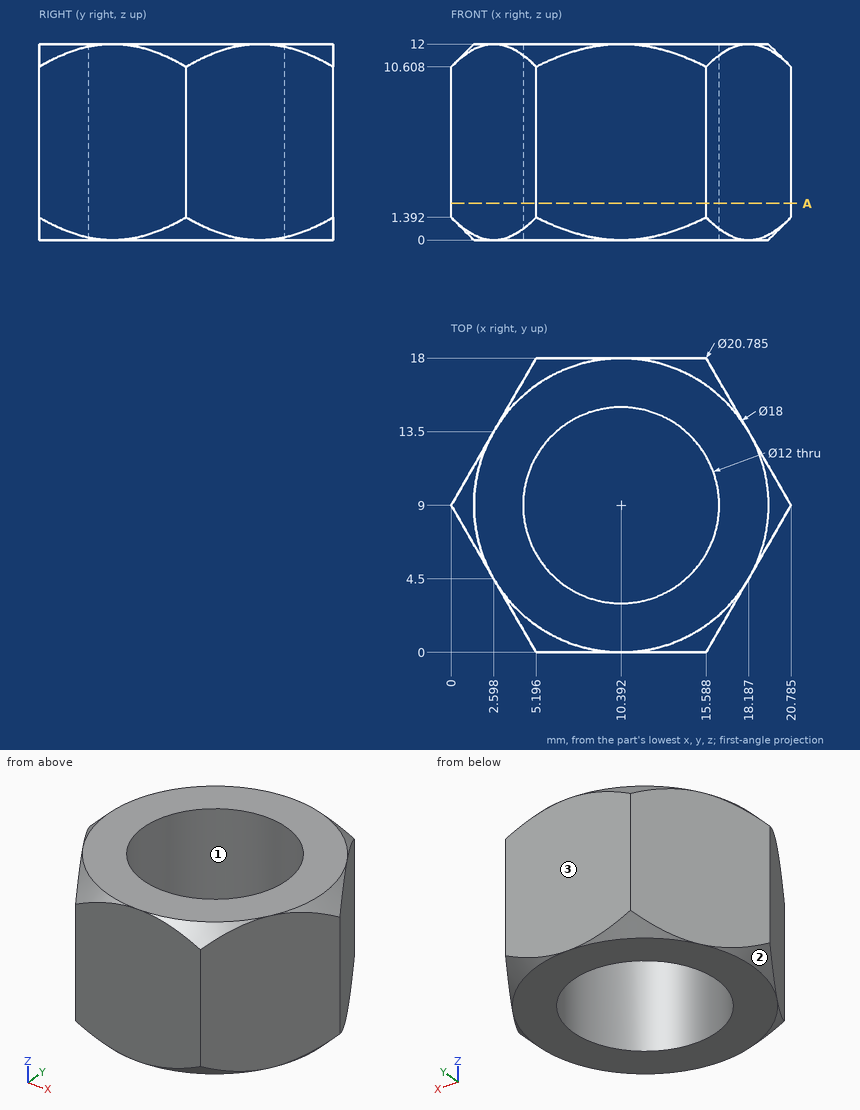
The figure shows three views and two pictorial views of one solid part (mm, origin at its lowest corner). Answer the questions. Give positions to 0.01 mm unless a question says otherwise; leave off trailing zeros. Loops run counter-clockwise (first coordinate to the right, second up) from the corner with the lowest first, then second, coordinate; pieces in that order, holes last. Notation, with made-up numbers: (30, 89.5) - (49, 89.5) arc R26 cw to (49, 127.5) - close; hole circle Ø1 at (84, -17). An arc over 180 degrees is marked (long way). Use one line per item in the form item = value.
1. The mould has two halves that part along Y. Classify the marked faces 1, 2 and 3: pulls with the +Y half, pulls with the -Y half, needs draft (parallel to the pull), parting line crosses it, or undercut.
Calculated:
face_1 = undercut
face_2 = parting line crosses it
face_3 = pulls with the +Y half
2. Section A-A on z = 2.25 is taken. Give the vertices of the cut face in (x, y) (1 decimal).
Calculated:
outline = (0, 9) - (5.2, 0) - (15.6, 0) - (20.8, 9) - (15.6, 18) - (5.2, 18) - close; hole circle Ø12 at (10.4, 9)
3. Find the intervals of material crossed by line 1 along Y through (x, z) = (10.25, 10); line 2 along Y through (x, z) = (9.5, 10); line 3 along X through (y, z) = (10.5, 11.5) (1 decimal), in increasing order. Write a range as [from, to].
Calculated:
line_1 = [0, 3], [15, 18]
line_2 = [0, 3.07], [14.93, 18]
line_3 = [1, 4.6], [16.2, 19.8]
4. Given pin 1 Ø2 at (x, z) = (10.5, 5) entering from -Y; pin 2 Ø3 at (y, z) = (13.5, 3) entering from -X; pin 3 Ø9.5 at (x, y) = (10.39, 9) entering from +Z; pin 4 Ø1.5 at (y, z) = (6.5, 7) entering from -X, each flat-ended and moving along its own axis, determine where each tip first touches the part or whether it passes through.
Calculated:
pin_1 = 0
pin_2 = 1.73
pin_3 = through
pin_4 = 1.01
